Part model, mm, in its own coordinate system. Face numbers are marked on the shaded views. A direction names the side the tool comes from. Round coordinates to 2 decimals unless told otherwise and drop trailing zeros. Order: outer loops, then holes, each group sorted by start corner. A loop starts at its lowest first (then second) coordinate and runs counter-clockwise, first axis right, second up. Notation, with made-up numbers: (22, 66) - (63, 66) arc R22 ccw to (63, 82) - close; hole circle Ø4 at (-15.75, -17.5). An arc over 180 degrees is marked (long way). Answer as a JSON object with one key per item and string values.
Autodesk Inventor part; units mm, degrees
ref_plane "Work Plane1" through (0, 3, 0) normal (0, -1, 0) x (1, 0, 0)
ref_plane "Work Plane2" through (0, 17, 0) normal (0, -1, 0) x (1, 0, 0)
ref_plane "YZ Plane" through (0, 0, 0) normal (1, 0, 0) x (0, 1, 0)
sketch "Sketch1" plane through (0, 0, 0) normal (0, 1, 0) x (-1, 0, 0)
  line L0 (6, 11.5) -> (-6, 11.5)
  line L1 (-6, 11.5) -> (-6, -11.5)
  line L2 (-6, -11.5) -> (6, -11.5)
  line L3 (6, -11.5) -> (6, 11.5)
  point P0 (0, 0)
  point P1 (6, 0)
  point P2 (0, 11.5)
  dimension "d0" = 23
  dimension "d1" = 12
extrude "Extrusion1" add sketch "Sketch1" along normal blind 25
sketch "Sketch2" plane through (-6, 0, 11.5) normal (0, 0, 1) x (1, 0, 0)
  line L0 (0, 23) -> (12, 23)
  line L1 (12, 23) -> (12, 21)
  line L2 (12, 21) -> (0, 21)
  line L3 (0, 21) -> (0, 23)
  line L4 (0, 0) -> (0, 25)
  line L5 (12, 0) -> (12, 25)
  line L6 (0, 0) -> (12, 0)
  point P0 (6, 0)
  dimension "d4" = 2
  dimension "d5" = 21
extrude "Extrusion2" add sketch "Sketch2" along normal blind 4.25 and the other way blind 27.25 contours L0 L1 L2 L3
sketch "Sketch3" plane through (0, 25, 0) normal (0, 1, 0) x (1, 0, 0)
  circle A0 centre (0, -5.5) radius 6
  circle A1 centre (0, 0.5) radius 3
  line L0 (-6, 11.5) -> (-6, -11.5)
  line L1 (6, -11.5) -> (6, 11.5)
  line L2 (-6, -11.5) -> (6, -11.5)
  line L3 (-6, 3.5) -> (6, 3.5) construction
  line L4 (-3, 0.5) -> (-3, -0.3038)
  line L5 (3, 0.5) -> (3, -0.3038)
  point P0 (0, 0)
  point P1 (0, -11.5)
  dimension "d10" = 12
  dimension "d11" = 6
  dimension "d12" = 15
extrude "Extrusion3" add sketch "Sketch3" along normal blind 5 contours A0 A1 | A0 A1 L5 | A1 A0 | A0 A1 | A0 L4 A1
sketch "Sketch4" plane through (0, 30, 0) normal (0, 1, 0) x (1, 0, 0)
  circle A0 centre (0, -5.5) radius 2.5
  arc A1 (-3, -0.3038) -> (3, -0.3038) centre (0, -5.5) ccw
  point P0 (0, 0)
  dimension "d15" = 5
extrude "Extrusion4" add sketch "Sketch4" along normal blind 4.5
sketch "Sketch5" plane through (-6, 0, 11.5) normal (0, 0, 1) x (1, 0, 0)
  line L0 (3.5, 2) -> (8.5, 2)
  line L1 (8.5, 2) -> (8.5, 0)
  line L2 (8.5, 0) -> (3.5, 0)
  line L3 (3.5, 0) -> (3.5, 2)
  line L4 (0, 0) -> (12, 0)
  circle A0 centre (4.5, 1) radius 1
  circle A1 centre (7.5, 1) radius 1
  circle A2 centre (6, 1) radius 1
  point P0 (6, 0)
  point P1 (6, 0)
  point P2 (6, 0)
  point P3 (6, 0)
  dimension "d18" = 5
  dimension "d19" = 2
extrude "Extrusion5" add sketch "Sketch5" along normal blind 5 contours A0 A2 | A2 A1 A0 | A0 A2 | A1 A2 | A2 A1
ref_plane "Work Plane1" through (0, 3, 0) normal (0, -1, 0) x (1, 0, 0)
ref_plane "Work Plane2" through (0, 17, 0) normal (0, -1, 0) x (1, 0, 0)
split_face "Split1"
split_face "Split2"
sketch "Sketch6" plane through (-6, 23, 11.5) normal (0, 1, 0) x (1, 0, 0)
  circle A0 centre (6, -2.5) radius 1
  line L0 (12, -4.25) -> (0, -4.25)
  line L1 (0, 0) -> (12, 0)
  point P0 (6, 11.5)
  point P1 (6, -4.25)
  dimension "d24" = 2
  dimension "d25" = 1.5
extrude "Extrusion6" cut sketch "Sketch6" against normal up to surface (2 mm away)
sketch "Sketch7" plane through (-6, 23, -11.5) normal (0, 1, 0) x (1, 0, 0)
  circle A0 centre (6, 2.5) radius 1
  line L0 (0, 4.25) -> (12, 4.25)
  line L1 (12, 0) -> (0, 0)
  point P0 (6, -11.5)
  point P1 (6, 4.25)
  dimension "d28" = 2
  dimension "d29" = 1.5
extrude "Extrusion7" cut sketch "Sketch7" against normal up to surface (2 mm away)
equation "\"d0\" = servo_A"
equation "\"d1\" = servo_B"
equation "\"d2\" = servo_F + servo_E + servo_J"
equation "\"d4\" = servo_F"
equation "\"d5\" = servo_E"
equation "\"d6\" = -0.5 * servo_A + 0.5 * servo_D"
equation "\"d7\" = d6 + servo_A"
equation "\"d10\" = servo_B"
equation "\"d11\" = servo_N"
equation "\"d12\" = servo_I"
equation "\"d13\" = -servo_F + servo_C - servo_E - servo_J"
equation "\"d15\" = servo_G"
equation "\"d16\" = servo_O - servo_C"
equation "\"d18\" = servo_K"
equation "\"d24\" = servo_H"
equation "\"d25\" = servo_L"
equation "\"d28\" = servo_H"
equation "\"d29\" = servo_L"
equation "\"servo_A\" = 23"
equation "\"servo_B\" = 12"
equation "\"servo_C\" = 30"
equation "\"servo_D\" = 31.5"
equation "\"servo_E\" = 21"
equation "\"servo_F\" = 2"
equation "\"servo_G\" = 5"
equation "\"servo_H\" = 2"
equation "\"servo_I\" = 15"
equation "\"servo_J\" = 2"
equation "\"servo_K\" = 5"
equation "\"servo_L\" = 1.5"
equation "\"servo_M\" = 5"
equation "\"servo_N\" = 6"
equation "\"servo_O\" = 34.5"
equation "\"servo_P\" = 33"
properties part number "TP-MG92B"
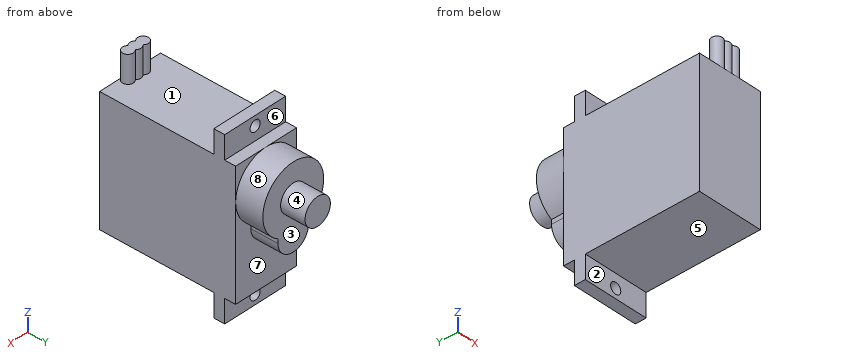
Item 1: Probe L1, parallel to Z at x = 0, y = 21.9; L2, parallel to X at y = 22.55, z = 14; L3, parallel to Y at x = 1, z = 10.5. List the from-to ranges inside material, lowest first. Write a range as from..to.
Taken from the geometry:
{"L1": "-15.75..-15, -13..13, 15..15.75", "L2": "-6..-1, 1..6", "L3": "0..30"}
Item 2: Cut at D-D (x = 4). Write the cut outline in (y, z).
Taken from the geometry:
{"outline": "(0, -11.5) - (21, -11.5) - (21, -15.75) - (23, -15.75) - (23, -11.5) - (25, -11.5) - (25, 1.03) - (30, 1.03) - (30, 9.97) - (25, 9.97) - (25, 11.5) - (23, 11.5) - (23, 15.75) - (21, 15.75) - (21, 11.5) - (0, 11.5) - close"}
Item 3: Cut at C-C (y = 1). Write the cut outline in (x, z), plus the area to 3 significant figures.
Taken from the geometry:
{"outline": "(-6, -11.5) - (6, -11.5) - (6, 11.5) - (2.5, 11.5) - (2.5, 16.5) - (-2.5, 16.5) - (-2.5, 11.5) - (-6, 11.5) - close", "area": "301 mm2"}
Item 4: Cut at B-B (z = 14). Write the cut outline in (x, y).
Taken from the geometry:
{"outline": "(-6, 21) - (-1, 21) - (-1, 23) - (-6, 23) - close; (-0.75, 0.34) arc R1 ccw to (0.75, 0.34) arc R1 ccw (long way) to (0.75, 1.66) arc R1 ccw to (-0.75, 1.66) arc R1 ccw (long way) to start; (1, 21) - (6, 21) - (6, 23) - (1, 23) - close"}
Item 5: Cut at A-A (z = -14). Write the cut outline in (x, y), plus the area to 3 significant figures.
Taken from the geometry:
{"outline": "(-6, 21) - (-1, 21) - (-1, 23) - (-6, 23) - close; (1, 21) - (6, 21) - (6, 23) - (1, 23) - close", "area": "20.0 mm2"}
Item 6: Drop flat-ended pins along their axis: P1, Ø2.5, axis at x = 0, z = 14, coming from the +Y side; P2, Ø5, axis at x = -1.5, z = 9.5, coming from the +Y side; P3, Ø1.5, axis at x = 0, z = -5.5, coming from the +Y side; P4, Ø1.5, axis at x = -4.5, y = 22.5, coming from the +Z side. Give the stop position or say it passes through.
Taken from the geometry:
{"P1": "y = 23", "P2": "y = 34.5", "P3": "y = 25", "P4": "z = 15.75"}
Item 7: Tool access for the marked faces 5, 6, 7 and 8: list every direction of +Z, -Z, +X, -X, +Y, -Y with a clear straight run to the whole face (end or side of a thin tool).
Taken from the geometry:
{"face 5": "-Z, +X, -X, -Y", "face 6": "+Z, +X, -X, +Y", "face 7": "-Z, +Y", "face 8": "+Y"}
Item 8: Two-plate mould, pull along Y, no slides. Class the marked faces 1, 2, 3 and 4: pulls with the +Y half, pulls with the -Y half, needs draft (parallel to the pull), parting line crosses it, or undercut.
Taken from the geometry:
{"face 1": "undercut", "face 2": "pulls with the -Y half", "face 3": "pulls with the +Y half", "face 4": "needs draft"}
